Geometry check sheet. Reference: the model listing, model coordinates, mm. A direction names the side the tool comes from. Round coordinates to 2 decimals unless told otherwise and drop trailing zeros. Loops run counter-clockwise (first coordinate to the right, second up) from the corner with the lowest first, then second, coordinate; pieces in that order, holes last. Notation, with made-up numbers: (-34, 85.5) -> (-28, 85.5) arc R13 ccw to (-28, 100.5) -> close; hole circle Ø3 at (-21.5, -1). An arc over 180 degrees is marked (long way). Use one line per item in the form item = value.
from build123d import *

# Parameters (mm, degrees)
SKETCH1_R           = 12.5
BOSS_EXTRUDE1_DEPTH = 61
SKETCH2_R           = 3.5
BOSS_EXTRUDE2_DEPTH = 2.5
SKETCH3_R           = 2
BOSS_EXTRUDE3_DEPTH = 1.5
BOSS_EXTRUDE4_DEPTH = 8
SKETCH5_R           = 1.5
CUT_EXTRUDE1_DEPTH  = 3


with BuildPart() as part:
    # Sketch1 → Boss-Extrude1 (new body)
    with BuildSketch(Plane(origin=(0, 0, 0), x_dir=(1, 0, 0), z_dir=(0, 1, 0))):
        with Locations(Location((0, 0, 0), (0, 0, 90))):
            Circle(SKETCH1_R)
    extrude(amount=BOSS_EXTRUDE1_DEPTH)

    # Sketch2 → Boss-Extrude2 (add)
    with BuildSketch(Plane(origin=(0, 61, 0), x_dir=(1, 0, 0), z_dir=(0, 1, 0))):
        with Locations(Location((0, 0, 0), (0, 0, 270))):
            Circle(SKETCH2_R)
    extrude(amount=BOSS_EXTRUDE2_DEPTH)

    # Sketch3 → Boss-Extrude3 (add)
    with BuildSketch(Plane(origin=(0, 63.5, 0), x_dir=(1, 0, 0), z_dir=(0, 1, 0))):
        with Locations(Location((0, 0, 0), (0, 0, 270))):
            Circle(SKETCH3_R)
    extrude(amount=BOSS_EXTRUDE3_DEPTH)

    # Sketch4 → Boss-Extrude4 (add)
    with BuildSketch(Plane(origin=(0, 65, 0), x_dir=(1, 0, 0), z_dir=(0, 1, 0))):
        with BuildLine():
            Line((-1.322876, 1.5), (1.322876, 1.5))
            ThreePointArc((1.322876, 1.5), (0, -2), (-1.322876, 1.5))
        make_face()
    extrude(amount=BOSS_EXTRUDE4_DEPTH)

    # Sketch5 → Cut-Extrude1 (cut)
    with BuildSketch(Plane(origin=(0, 61, 0), x_dir=(1, 0, 0), z_dir=(0, 1, 0))):
        with Locations(Location((0, 8.6, 0), (0, 0, 270))):
            Circle(SKETCH5_R)
        with Locations(Location((0, -8.6, 0), (0, 0, 270))):
            Circle(SKETCH5_R)
    extrude(amount=-CUT_EXTRUDE1_DEPTH, mode=Mode.SUBTRACT)


solid = part.part
1. Section check A-A (z = 0). Record the boundary of the cut face in (x, y).
Return value:
outline = (-12.5, 0) -> (12.5, 0) -> (12.5, 61) -> (3.5, 61) -> (3.5, 63.5) -> (2, 63.5) -> (2, 73) -> (-2, 73) -> (-2, 63.5) -> (-3.5, 63.5) -> (-3.5, 61) -> (-12.5, 61) -> close
2. Section check B-B (y = 67.5). Record the boundary of the cut face in (x, z), then the cut area to 3 significant figures.
Return value:
outline = (-1.32, -1.5) -> (1.32, -1.5) arc R2 ccw (long way) to start
area = 11.7 mm2
3. Section check C-C (z = 8.6). Record the boundary of the cut face in (x, y).
Return value:
outline = (-9.07, 0) -> (9.07, 0) -> (9.07, 61) -> (1.5, 61) -> (1.5, 58) -> (-1.5, 58) -> (-1.5, 61) -> (-9.07, 61) -> close
4. Mould release check, pull along Z, two halves, no side actions. Record for faces 3 (the flat face through (0, 0, 0)), 4 (the flat face through (0, 69, -1.5)), 5 (the cylindrical face through (-3.755, 30.073, -11.923)), 6 (the flat face through (0, 58, 9)): released by +Z, released by -Z, zero draft, split by the parting line, or undercut.
Return value:
face_3 = zero draft
face_4 = released by -Z
face_5 = split by the parting line
face_6 = undercut
5. Material ranges on line 1 along Y through (x, z) = (1.25, -9); line 2 along Y through (x, z) = (6.5, 4.75); line 3 along X through (y, z) = (33.5, -0.25), recorded low to high.
Return value:
line_1 = 0 to 58
line_2 = 0 to 61
line_3 = -12.5 to 12.5
6. Gauge pin test, flat ends, axial feed: pin 1 (1.5 mm diameter, centred on x = 7.5, z = -7.5, fed in from +Y); pin 2 (1 mm diameter, centred on x = 3, y = 54.5, fed in from +Z); pin 3 (4 mm diameter, centred on y = 53.5, z = 3, fed in from +X). Record the tip position at first contact, or that the pin passes through.
Return value:
pin_1 = 61
pin_2 = 12.25
pin_3 = 12.46
7. Section check D-D (x = -4.25). Record the boundary of the cut face in (y, z).
Return value:
outline = (0, -11.76) -> (61, -11.76) -> (61, 11.76) -> (0, 11.76) -> close
8. Tool access check on faces 1 (the flat face through (-2, 63.5, 2)), 2 (the flat face through (0, 73, 0)). Record the directions out of +Z, -Z, +X, -X, +Y, -Y that give a thin tool (end or side, any length) a straight path to the whole face; none if there is none.
Return value:
face_1 = +Y
face_2 = +Z, -Z, +X, -X, +Y
